Build history of the part. All positions in model axes, mm. Face numbers are marked on the shaded views. A direction names the side the tool comes from. Round coordinates to 2 decimals unless told otherwise and drop trailing zeros. Write each loop counter-clockwise with the first axis right and the second up, starting at its lowest first coordinate (ties: lowest second). Pieces come first, ordered by that corner, then holes. Notation, with made-up numbers: M -22.75,47 L 7.25,47 A10 ccw 7.25,63 Z; hole C -19,86.25 d2. An arc over 180 degrees is marked long. One line per item, written item: value. Start each with the question number.
```python
from build123d import *

# Parameters (mm, degrees)
SKETCH1_W            = 35.55
SKETCH1_H            = 35.55
SKETCH1_W_2          = 25.55
SKETCH1_H_2          = 25.55
BOSS_EXTRUDE1_DEPTH  = 25
SKETCH2_R            = 1.25
CUT_EXTRUDE1_DEPTH   = 4
SKETCH3_W            = 20
SKETCH3_H            = 22
SKETCH3_R            = 4
BOSS_EXTRUDE2_DEPTH  = 5
FILLET1_R            = 10
FILLET1_OF_MIRROR2_R = 10


with BuildPart() as part:
    # Sketch1 → Boss-Extrude1 (new, symmetric)
    with BuildSketch(Plane.XY):
        Rectangle(SKETCH1_W, SKETCH1_H)
        Rectangle(SKETCH1_W_2, SKETCH1_H_2, mode=Mode.SUBTRACT)
    extrude(amount=BOSS_EXTRUDE1_DEPTH, both=True)

    # Sketch2 → Cut-Extrude1 (cut, symmetric)
    with BuildSketch(Plane.ZY.offset(17.775)):
        with Locations((-15.6, -14.775)):
            Circle(SKETCH2_R)
        with Locations((15.6, -14.775)):
            Circle(SKETCH2_R)
        with Locations((-15.6, -8.375)):
            Circle(SKETCH2_R)
        with Locations((15.6, -8.375)):
            Circle(SKETCH2_R)
        with Locations((-15.6, -1.975)):
            Circle(SKETCH2_R)
        with Locations((15.6, -1.975)):
            Circle(SKETCH2_R)
        with Locations((-15.6, 4.425)):
            Circle(SKETCH2_R)
        with Locations((15.6, 4.425)):
            Circle(SKETCH2_R)
        with Locations((-15.6, 10.825)):
            Circle(SKETCH2_R)
        with Locations((15.6, 10.825)):
            Circle(SKETCH2_R)
    extrude(amount=CUT_EXTRUDE1_DEPTH, both=True, mode=Mode.SUBTRACT)

    # Sketch3 → Boss-Extrude2 (add)
    with BuildSketch(Plane.XY.offset(25)):
        with Locations((27.775, 0)):
            Rectangle(SKETCH3_W, SKETCH3_H)
        with Locations((27.775, 0)):
            Circle(SKETCH3_R, mode=Mode.SUBTRACT)
    boss_extrude2 = extrude(amount=-BOSS_EXTRUDE2_DEPTH)

    # Fillet1
    # the kernel refuses this fillet: 10 mm, written as the material it adds along each edge
    with BuildSketch(Plane(origin=(17.775, -11, 25), x_dir=(0, -1, 0), z_dir=(0, 0, -1))) as fillet1_piece_1:
        with BuildLine():
            CenterArc((10, -9.465694639), FILLET1_R, 108.814181852, 71.185818148)
            Line((0, -9.465694639), (-0.2, -9.465694639))
            Line((-0.2, -9.465694639), (-0.2, 0))
            Line((-0.2, 0), (0, 0.2))
            ThreePointArc((0, 0.2), (3.3875, 0.2), (6.7105, 0.189313893))
            Line((6.7105, 0.189313893), (6.775, 0))
        make_face()
    extrude(amount=5)
    with BuildSketch(Plane(origin=(17.775, 11, 25), x_dir=(0, 1, 0), z_dir=(0, 0, -1))) as fillet1_piece_2:
        with BuildLine():
            CenterArc((10, 9.465694639), FILLET1_R, 180, 71.185818148)
            Line((0, 9.465694639), (-0.2, 9.465694639))
            Line((-0.2, 9.465694639), (-0.2, 0))
            Line((-0.2, 0), (0, -0.2))
            ThreePointArc((0, -0.2), (3.3875, -0.2), (6.7105, -0.189313893))
            Line((6.7105, -0.189313893), (6.775, 0))
        make_face()
    extrude(amount=5)

    # Mirror2: Boss-Extrude2 across plane
    add(boss_extrude2.mirror(Plane.XY))

    # Fillet1 of Mirror2
    # the kernel refuses this fillet: 10 mm, written as the material it adds along each edge
    with BuildSketch(Plane(origin=(17.775, -11, -25), x_dir=(0, -1, 0), z_dir=(0, 0, 1))) as fillet1_of_mirror2_piece_1:
        with BuildLine():
            CenterArc((10, 9.465694639), FILLET1_OF_MIRROR2_R, 180, 71.185818148)
            Line((0, 9.465694639), (-0.2, 9.465694639))
            Line((-0.2, 9.465694639), (-0.2, 0))
            Line((-0.2, 0), (0, -0.2))
            ThreePointArc((0, -0.2), (3.3875, -0.2), (6.7105, -0.189313893))
            Line((6.7105, -0.189313893), (6.775, 0))
        make_face()
    extrude(amount=5)
    with BuildSketch(Plane(origin=(17.775, 11, -25), x_dir=(0, 1, 0), z_dir=(0, 0, 1))) as fillet1_of_mirror2_piece_2:
        with BuildLine():
            CenterArc((10, -9.465694639), FILLET1_OF_MIRROR2_R, 108.814181852, 71.185818148)
            Line((0, -9.465694639), (-0.2, -9.465694639))
            Line((-0.2, -9.465694639), (-0.2, 0))
            Line((-0.2, 0), (0, 0.2))
            ThreePointArc((0, 0.2), (3.3875, 0.2), (6.7105, 0.189313893))
            Line((6.7105, 0.189313893), (6.775, 0))
        make_face()
    extrude(amount=5)


solid = part.part
```
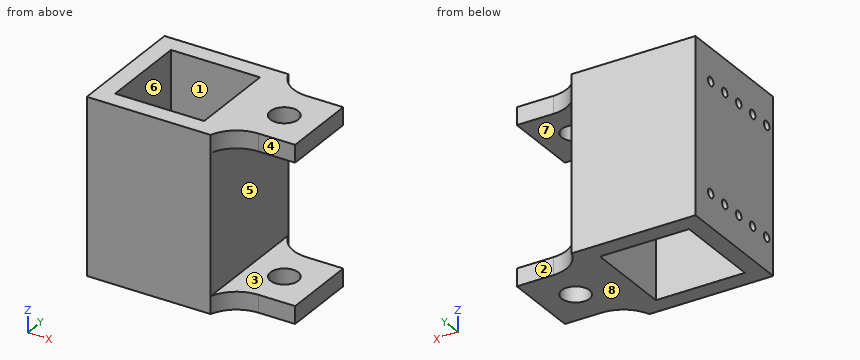
Item 1: Drop flat-ended pins along their axis: pin 1 (9 mm diameter, centred on x = 27.775, y = 0, fed in from -Z); pin 2 (1.2 mm diameter, centred on y = -8, z = -15.5, fed in from -X) (3 decimals); pin 3 (1 mm diameter, centred on y = 2.5, z = 19, fed in from +X) (3 decimals); pin 4 (2.5 mm diameter, centred on x = 34, z = -22, fed in from +Y). Give the stop position or say it passes through.
Item 2: Cut at D-D, the plane x = 10. Write the cut outline in (y, z) (3 decimals).
Item 3: Two-plate mould, pull along Z, no slides. Class the marked faces 5, 6, 7 and 8: pulls with the +Z half, pulls with the -Z half, needs draft (parallel to the pull), parting line crosses it, or undercut.
Item 4: Cut at C-C, the plane y = 0. Write the cut outline in (x, z) (3 decimals).
Item 5: Drill centre lines: line 1 (Y direction, x = -16, z = 15.6) (3 decimals); line 2 (Y direction, x = -6, z = 15) (3 decimals); line 3 (Z direction, x = 33, y = -3). Where is each one in solid material? Low to high.
Item 6: Which spindle directions (+Z, -Z, +X, -X, +Y, -Y) get a long thin tool onto all of the face, cutting with end or side? Do the marked faces 1, 2, 3 and 4. Say none if no direction does.
Item 7: Cut at B-B, the plane z = -15.6. Write the cut outline in (x, y) (3 decimals), plus the area to 3 significant figures.
Item 8: Cut at A-A, the plane y = -5. Write the cut outline in (x, z) (3 decimals).
Computed values:
1. pin 1: stops at z = -25
1. pin 2: stops at x = -13.775
1. pin 3: stops at x = 17.775
1. pin 4: stops at y = 11
2. outline: M -17.775,-25 L -12.775,-25 L -12.775,25 L -17.775,25 Z; M 12.775,-25 L 17.775,-25 L 17.775,25 L 12.775,25 Z
3. face 5: undercut
3. face 6: needs draft
3. face 7: undercut
3. face 8: pulls with the -Z half
4. outline: M -17.775,-25 L -12.775,-25 L -12.775,25 L -17.775,25 Z; M 12.775,-25 L 23.775,-25 L 23.775,-20 L 17.775,-20 L 17.775,20 L 23.775,20 L 23.775,25 L 12.775,25 Z; M 31.775,-25 L 37.775,-25 L 37.775,-20 L 31.775,-20 Z; M 31.775,20 L 37.775,20 L 37.775,25 L 31.775,25 Z
5. line 1: y = -17.775 to -16.025, -13.525 to -9.625, -7.125 to -3.225, -0.725 to 3.175, 5.675 to 9.575, 12.075 to 17.775
5. line 2: y = -17.775 to -12.775, 12.775 to 17.775
5. line 3: z = -25 to -20, 20 to 25
6. face 1: +Z, -Z
6. face 2: +Z, -Z, +X, +Y
6. face 3: +X, +Y, -Y
6. face 4: +Z, -Z, +X, -Y
7. outline: M -17.775,-17.775 L 17.775,-17.775 L 17.775,17.775 L -17.775,17.775 L -17.775,12.075 L -13.775,12.075 L -13.775,9.575 L -17.775,9.575 L -17.775,5.675 L -13.775,5.675 L -13.775,3.175 L -17.775,3.175 L -17.775,-0.725 L -13.775,-0.725 L -13.775,-3.225 L -17.775,-3.225 L -17.775,-7.125 L -13.775,-7.125 L -13.775,-9.625 L -17.775,-9.625 L -17.775,-13.525 L -13.775,-13.525 L -13.775,-16.025 L -17.775,-16.025 Z; hole M -12.775,-12.775 L 12.775,-12.775 L 12.775,12.775 L -12.775,12.775 Z
7. area: 561 mm2
8. outline: M -17.775,-25 L -12.775,-25 L -12.775,25 L -17.775,25 Z; M 12.775,-25 L 37.775,-25 L 37.775,-20 L 17.775,-20 L 17.775,20 L 37.775,20 L 37.775,25 L 12.775,25 Z
